```python
from build123d import *

# Parameters (mm, degrees)
M3_GEWINDEBOHRUNG1_D     = 2.5
M3_GEWINDEBOHRUNG1_DEPTH = 5
M3_GEWINDEBOHRUNG1_TIP   = 0.751075774


with BuildPart() as part:
    # Skizze1 → Rotation1 (revolve)
    with BuildSketch(Plane.XY):
        Polygon((0, 3), (5, 3), (5, 1.5), (11, 1.5), (11, 0), (0, 0), align=None)
    revolve(axis=Axis((11, 0, 0), (-1, 0, 0)))

    # M3 Gewindebohrung1
    with Locations(Plane.ZY):
        with Locations((0, 0)):
            Hole(M3_GEWINDEBOHRUNG1_D / 2, depth=M3_GEWINDEBOHRUNG1_DEPTH)
            with Locations((0, 0, -(M3_GEWINDEBOHRUNG1_DEPTH + M3_GEWINDEBOHRUNG1_TIP / 2))):  # 118° drill point
                Cone(0, M3_GEWINDEBOHRUNG1_D / 2, M3_GEWINDEBOHRUNG1_TIP, mode=Mode.SUBTRACT)


solid = part.part
```
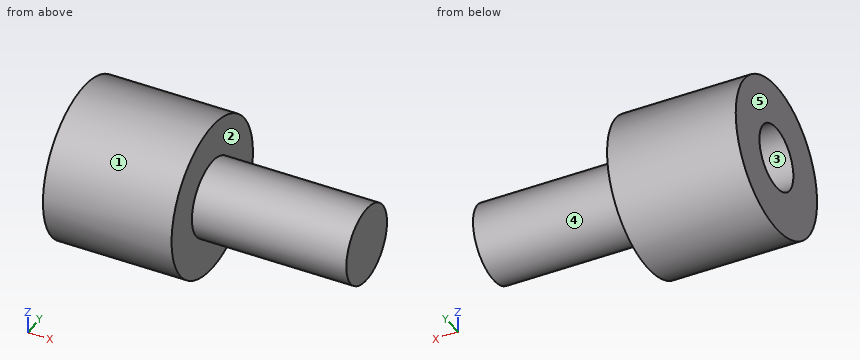
Work out the finished part from the listing and answer in its coordinate system (mm). Face numbers are marked on the shaded views. A direction names the side the tool comes from. Coordinates: 2 decimals unless noted, no trailing zeros. Write each loop counter-clockwise with the first axis right and the second up, starting at its lowest first coordinate (ties: lowest second). Pieces come first, ordered by that corner, then holes.
Q1. A cutting plane is placed at A-A, the plane x = 1.75. Give the vertices of the cut face in (y, z), then the cut area to 3 significant figures.
Q2. A cutting plane is placed at D-D, the plane z = -1.7. Give the vertices of the cut face in (x, y).
Q3. A cutting plane is placed at B-B, the plane x = 6. Give the vertices of the cut face in (y, z).
Q4. A cutting plane is placed at C-C, the plane y = 2.3. Give the vertices of the cut face in (x, z), then the cut area to 3 significant figures.
Q5. Determine the mould class of the marked faces 3, 4 and 5 for opening direction Y: released by +Y, released by -Y, zero draft, split by the parting line, or undercut.
Q6. Find the intervals of material crossed by line 1 (Z direction, x = 2.2, y = 0); line 2 (X direction, y = -1.6, z = 0.35), in increasing order.
Q7. This flat-tipped pin is pushed along its axis until it touches: pin 1 Ø1.5 at (y, z) = (0, 0) entering from -X. Where does it stop, or does it pass through?
Q8. Which of the six approach directions +Z, -Z, +X, -X, +Y, -Y give full straight-line access (tool end or side, diameter ignored) to the marked faces 1 and 2?
Findings below:
1. outline: circle Ø6 at (0, 0); hole circle Ø2.5 at (0, 0)
1. area: 23.4 mm2
2. outline: (0, -2.47) - (5, -2.47) - (5, 2.47) - (0, 2.47) - close
3. outline: circle Ø3 at (0, 0)
4. outline: (0, -1.93) - (5, -1.93) - (5, 1.93) - (0, 1.93) - close
4. area: 19.3 mm2
5. face 3: undercut
5. face 4: split by the parting line
5. face 5: zero draft
6. line 1: z = -3 to -1.25, 1.25 to 3
6. line 2: x = 0 to 5
7. pin 1: stops at x = 5.3
8. face 1: +X, -X
8. face 2: +X
